Answer from the drawing. Dimensions are ordinates in mm from the lowest x, y and z of the part. A direction names the side the tool comes from. Round coordinates to 2 decimals unless told otherwise and drop trailing zeros. Loops run counter-clockwise (first coordinate to the right, second up) from the corner with the lowest first, then second, coordinate; pieces in that order, holes last. Notation, with made-up numbers: M -14.75,21 L 1.25,21 A21 cw 1.25,45 Z; hole C -37,87.5 d2. An arc over 180 degrees is marked long. Write each question's results on one line, items separated by ' | '.
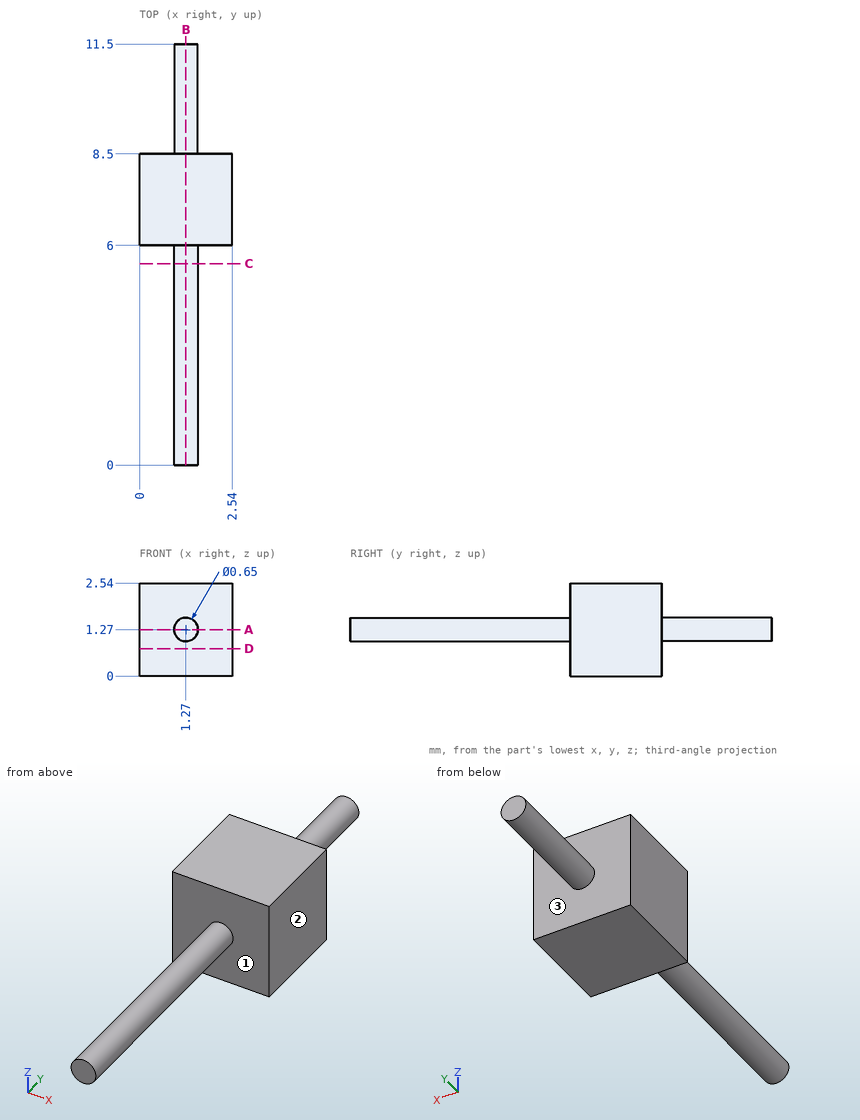
1. Find section B-B, the plane x = 1.27. Give the vertices of the cut face in (y, z) (3 decimals), then the cut area to 3 significant figures.
Completed:
outline: M 0,0.945 L 6,0.945 L 6,0 L 8.5,0 L 8.5,0.945 L 11.5,0.945 L 11.5,1.595 L 8.5,1.595 L 8.5,2.54 L 6,2.54 L 6,1.595 L 0,1.595 Z | area: 12.2 mm2
2. Find the intervals of material crossed by L1, parallel to Y at x = 2.3, z = 0.55; L2, parallel to X at y = 10.5, z = 1.3; L3, parallel to X at y = 2.75, z = 1.5, in increasing order.
Completed:
L1: y = 6 to 8.5 | L2: x = 0.95 to 1.59 | L3: x = 1.04 to 1.5
3. Find section C-C, the plane y = 5.5. Give the vertices of the cut face in (x, z) (3 decimals), then the cut area to 3 significant figures.
Completed:
outline: C 1.27,1.27 d0.65 | area: 0.332 mm2
4. Given P1, Ø1, axis at y = 2, z = 1, coming from the +X side (3 decimals), flat-ended and moving along its own axis, determine where the tip first touches the part or whether it passes through.
Completed:
P1: stops at x = 1.595
5. Find section A-A, the plane z = 1.27. Give the vertices of the cut face in (x, y) (3 decimals), then the cut area to 3 significant figures.
Completed:
outline: M 0,6 L 0.945,6 L 0.945,0 L 1.595,0 L 1.595,6 L 2.54,6 L 2.54,8.5 L 1.595,8.5 L 1.595,11.5 L 0.945,11.5 L 0.945,8.5 L 0,8.5 Z | area: 12.2 mm2
6. Find section D-D, the plane z = 0.75. Give the vertices of the cut face in (x, y).
Completed:
outline: M 0,6 L 2.54,6 L 2.54,8.5 L 0,8.5 Z
7. Which of the six approach directions +Z, -Z, +X, -X, +Y, -Y give full straight-line access (tool end or side, diameter ignored) to the marked faces 1, 2 and 3?
Completed:
face 1: -Y | face 2: +Z, -Z, +X, +Y, -Y | face 3: +Y
